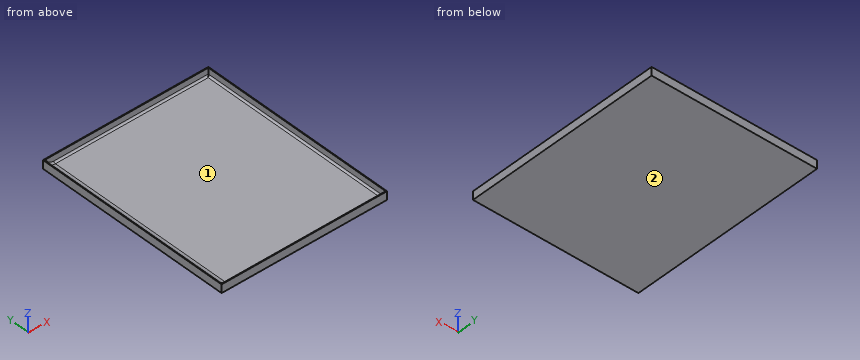
```python
from build123d import *

# Parameters (mm, degrees)
F0_W        = 200
F0_H        = 240
F1_DEPTH    = 10
F2_T        = -0.8
F3_T1_DEPTH = 238.4
F4_R        = 2


# Not quite as in the source:
# - a fillet or chamfer that OpenCascade refuses, or shapes differently, is made with other operations: its cross-section is extruded or revolved along the edge and cut away or added


with BuildPart() as f1:
    # F0 (on Top) → F1 (new body)
    with BuildSketch(Plane.XY):
        with Locations((9.3512600348, 8.6151771247)):
            Rectangle(F0_W, F0_H)
    extrude(amount=F1_DEPTH)

    # F2
    f2_openings = [f1.faces().sort_by_distance(p)[0] for p in [
        (9.35126, 8.615177, 10),
    ]]
    offset(amount=F2_T, openings=f2_openings)

    # F3: fillet of radius 12 on 1 edges, made by hand

    # F3_s2 → F3_t1 (join)
    with BuildSketch(Plane.XZ.offset(-127.8151771247)):
        with BuildLine():
            ThreePointArc((-89.8487399652, 10), (-85.609648497, 3.3766248085), (-78.1799782486, 0.8))
            Line((-78.1799782486, 0.8), (-89.8487399652, 0.8))
            Line((-89.8487399652, 0.8), (-89.8487399652, 10))
        make_face()
    extrude(amount=F3_T1_DEPTH)

    # F4
    f4_edges = [f1.edges().sort_by_distance(p)[0] for p in [
        (15.185641, 127.815177, 0.8),
        (15.185641, -110.584823, 0.8),
        (108.55126, 8.615177, 0.8),
        (-85.609648, 127.815177, 3.376625),
        (-85.609648, -110.584823, 3.376625),
    ]]
    fillet(f4_edges, radius=F4_R)


solid = f1.part
```
Could you check a few things on this model? Use its own coordinates, in mm. Face numbers are marked on the shaded views. Coordinates: 2 decimals unless noted, no trailing zeros. Write each loop counter-clockwise with the first axis right and the second up, starting at its lowest first coordinate (ties: lowest second). Pieces come first, ordered by that corner, then holes. Notation, with made-up numbers: (32.5, 48.5) -> (75.5, 48.5) arc R36 ccw to (75.5, 82.5) -> close; hole circle Ø5 at (-26.5, -35.5). An arc over 180 degrees is marked (long way). Return JSON: item names as keys, results as strings.
(1) I need wall thicknesses on L1, parallel to Y at x = -43.5, z = 2.5; L2, parallel to Z at x = 16, y = -95; L3, parallel to X at y = 6, z = 2.5. Which ranges of each line are inside material? Lowest first, please.
Numbers:
{"L1": "y = -111.38 to -110.56, 127.79 to 128.62", "L2": "z = 0 to 0.8", "L3": "x = -90.65 to -84.34, 108.53 to 109.35"}
(2) We'd pull the mould along X, two halves only. Please class the marked faces 1 and 2: +X half, -X half, draft (parallel to the pull), parting line (faces both ways), or undercut.
Numbers:
{"face 1": "undercut", "face 2": "draft"}
(3) Imagine slicing it at A-A, the plane x = -75. Please give me the cut outline in (y, z), then the cut area to 3 significant figures.
Numbers:
{"outline": "(-111.38, 0) -> (128.62, 0) -> (128.62, 10) -> (127.82, 10) -> (127.82, 2.8) arc R2 cw to (125.82, 0.8) -> (-108.58, 0.8) arc R2 cw to (-110.58, 2.8) -> (-110.58, 10) -> (-111.38, 10) -> close", "area": "208 mm2"}
(4) I'm going to push a flat-ended pin straight in: pin 1 (10 mm diameter, centred on x = 76, y = 40.5, fed in from +Z). Where does the tip first touch, or does it pass through?
Numbers:
{"pin 1": "stops at z = 0.8"}
(5) Imagine slicing it at B-B, the plane y = -33.5. Please give me the cut outline in (x, z).
Numbers:
{"outline": "(-90.65, 0) -> (109.35, 0) -> (109.35, 10) -> (108.55, 10) -> (108.55, 2.8) arc R2 cw to (106.55, 0.8) -> (-78.18, 0.8) arc R12 cw to (-89.85, 10) -> (-90.65, 10) -> close"}
